```python
from build123d import *

# Parameters (mm, degrees)
BOSS_EXTRUDE1_DEPTH          = 10
CONVERT_SOLID1_DEPTH         = 6
EDGE_FLANGE2_DEPTH           = 600
EDGE_FLANGE4_STRIP_CUT_DEPTH = 600
EDGE_FLANGE4_DEPTH           = 600
CUT_EXTRUDE2_DEPTH           = 952.374861111
CUT_EXTRUDE2_DEPTH_BACK      = 952.374861111


# Read off the part's stored shape, not the designer's step: Convert-Solid1
# Sheet-metal steps are written as plain solids
with BuildPart() as part:
    # Sketch1 → Boss-Extrude1 (new body)
    with BuildSketch(Plane(origin=(0, 0, 0), x_dir=(1, 0, 0), z_dir=(0, 1, 0))):
        Polygon((-192.279765905, 0), (-192.279765905, 237.5), (404.456147209, 300), (404.456147209, 0), (404.456147209, -300), (-192.279765905, -237.5), align=None)
    extrude(amount=BOSS_EXTRUDE1_DEPTH)

    # Convert-Solid1 outline → Convert-Solid1 (cut)
    with BuildSketch(Plane(origin=(0, 0, 0), x_dir=(1, 0, 0), z_dir=(0, 1, 0))):
        Polygon((-192.279765905, -237.5), (404.456147209, -300), (404.456147209, 300), (-192.279765905, 237.5), align=None)
    extrude(amount=CONVERT_SOLID1_DEPTH, mode=Mode.SUBTRACT)

    # Edge-Flange2 section (across the edge) → Edge-Flange2 (add)
    with BuildSketch(Plane(origin=(414.456147209, 10, 300), x_dir=(-0.9659258262890673, 0.25881904510252446, 0), z_dir=(0, 0, -1))):
        with BuildLine():
            Line((-4, 7.67326988), (-4, 187.930692048))
            Line((-4, 187.930692048), (0, 187.930692048))
            Line((0, 187.930692048), (0, 7.67326988))
            ThreePointArc((0, 7.67326988), (2.066466597, 1.58565559), (7.411809549, -1.985988383))
            Line((7.411809549, -1.985988383), (9.659258263, -2.588190451))
            Line((9.659258263, -2.588190451), (8.623982082, -6.451893756))
            Line((8.623982082, -6.451893756), (6.376533369, -5.849691688))
            ThreePointArc((6.376533369, -5.849691688), (-1.106946764, -0.849390126), (-4, 7.67326988))
        make_face()
    extrude(amount=EDGE_FLANGE2_DEPTH)

    # Edge-Flange4 strip (across the edge) → Edge-Flange4 strip cut (cut)
    with BuildSketch(Plane(origin=(463.09618947, 191.527109002, 300), x_dir=(-0.9961946980917449, 0.0871557427476667, 0), z_dir=(0, 0, -1))):
        Polygon((-10.038642938, 33.896891256), (-3.787308542, -1.556187852), (0.15192247, -0.861595141), (-6.099411926, 34.591483967), align=None)
    extrude(amount=EDGE_FLANGE4_STRIP_CUT_DEPTH, mode=Mode.SUBTRACT)

    # Edge-Flange4 section (across the edge) → Edge-Flange4 (add)
    with BuildSketch(Plane(origin=(463.09618947, 191.527109002, 300), x_dir=(-0.9961946980917449, 0.0871557427476667, 0), z_dir=(0, 0, -1))):
        with BuildLine():
            Line((-4, 0.874886635), (-4, 412.850045346))
            Line((-4, 412.850045346), (0, 412.850045346))
            Line((0, 412.850045346), (0, 0.874886635))
            ThreePointArc((0, 0.874886635), (0.038053019, 0.003329208), (0.15192247, -0.861595141))
            Line((0.15192247, -0.861595141), (-3.787308542, -1.556187852))
            ThreePointArc((-3.787308542, -1.556187852), (-3.946725773, -0.345293763), (-4, 0.874886635))
        make_face()
    extrude(amount=EDGE_FLANGE4_DEPTH)

    # Sketch22 → Cut-Extrude2 (cut, two sides: drawn at the far end of the back side and taken through both)
    with BuildSketch(Plane(origin=(442.9492869, -38.753041121, 0), x_dir=(0, 0, 1), z_dir=(-0.9961946980917449, 0.08715574274766662, 0)).offset(-CUT_EXTRUDE2_DEPTH_BACK)):
        Polygon((300, 232.03466952), (196.591479546, 525.272945681), (153.798650158, 525.272945681), (87.551647761, 644.009828231), (302.699803465, 645.121208779), (304.833664863, 232.03466952), align=None)
        Polygon((-300, 232.03466952), (-196.591479546, 525.272945681), (-153.798650158, 525.272945681), (-87.551647761, 644.009828231), (-302.699803465, 645.121208779), (-304.833664863, 232.03466952), align=None)
    extrude(amount=CUT_EXTRUDE2_DEPTH + CUT_EXTRUDE2_DEPTH_BACK, mode=Mode.SUBTRACT)


solid = part.part
```
The listing builds one solid part. Answer for the finished solid, in the listing's coordinates (mm). Round coordinates to 2 decimals unless told otherwise and drop trailing zeros. Loops run counter-clockwise (first coordinate to the right, second up) from the corner with the lowest first, then second, coordinate; pieces in that order, holes last.
1) For a pull along Y with two mould halves and no side action, classify faces 1 (the face through (443.195, 101.799, 4.2)), 2 (the face through (438, 92, 300)), 3 (the face through (495.85, 542.66, -121.14)) as released by +Y, released by -Y, zero draft, split by the parting line, or undercut.
Outcome:
face 1: released by -Y
face 2: zero draft
face 3: released by +Y
2) A cutting plane is placed at A-A on z = -49. Determine the outline of the cut face in (x, y), plus the area to 3 significant figures.
Outcome:
outline: (-192.28, 6) - (406.78, 6) arc R14 ccw to (420.31, 16.38) - (466.73, 189.65) arc R14 ccw to (467.16, 192.05) - (503.06, 602.46) - (499.08, 602.81) - (463.17, 192.4) arc R10 cw to (462.87, 190.68) - (416.44, 17.41) arc R10 cw to (406.78, 10) - (-192.28, 10) - close
area: 4,830 mm2
3) Consider line 1 (Y direction, x = -143, z = -197.5); line 2 (X direction, y = 206, z = 126); line 3 (X direction, y = 385.5, z = -128.5). Determine where each line is inside the solid, lowest interval first.
Outcome:
line 1: y = 6 to 10
line 2: x = 464.36 to 468.38
line 3: x = 480.07 to 484.08
4) Given P1, Ø2, axis at y = 101, z = -144, coming from the +X side; P2, Ø8, axis at x = 132, z = 127.5, coming from the +Y side; P3, Ø2, axis at y = 142, z = -67, coming from the +X side, each flat-ended and moving along its own axis, determine where each tip first touches the part or whether it passes through.
Outcome:
P1: stops at x = 443.25
P2: stops at y = 10
P3: stops at x = 454.23
5) A cutting plane is placed at B-B on z = -187. Determine the outline of the cut face in (x, y), plus the area to 3 significant figures.
Outcome:
outline: (-192.28, 6) - (406.78, 6) arc R14 ccw to (420.31, 16.38) - (466.73, 189.65) arc R14 ccw to (467.16, 192.05) - (492.71, 484.17) - (488.73, 484.52) - (463.17, 192.4) arc R10 cw to (462.87, 190.68) - (416.44, 17.41) arc R10 cw to (406.78, 10) - (-192.28, 10) - close
area: 4,360 mm2
6) A cutting plane is placed at C-C on x = -95. Determine the outline of the cut face in (y, z), plus the area to 3 significant figures.
Outcome:
outline: (6, -247.69) - (10, -247.69) - (10, 247.69) - (6, 247.69) - close
area: 1,980 mm2
7) A cutting plane is placed at D-D on y = 518. Determine the outline of the cut face in (x, z), plus the area to 3 significant figures.
Outcome:
outline: (491.66, -135.05) - (495.67, -134.85) - (495.67, 134.85) - (491.66, 135.05) - close
area: 1,080 mm2
